Verification items for the finished model (mm, model axes). Give positions to 0.01 mm unless a question says otherwise; leave off trailing zeros. Write each loop counter-clockwise with the first axis right and the second up, starting at its lowest first coordinate (ties: lowest second). Pieces come first, ordered by that corner, then holes.
from build123d import *

# Parameters (mm, degrees)
EXTRUDE_1_DEPTH     = 3
SKETCH_3_R          = 1.25
SKETCH_3_R_2        = 30
SKETCH_3_R_3        = 1.5
CUT_EXTRUDE_1_DEPTH = 3
CUT_EXTRUDE_2_DEPTH = 3
SKETCH_5_R          = 1.25
CUT_EXTRUDE_3_DEPTH = 10


with BuildPart() as part:
    # 草图2 → 凸台-拉伸1 (new body)
    with BuildSketch(Plane(origin=(0, 5, 0), x_dir=(1, 0, 0), z_dir=(0, 1, 0))):
        with BuildLine():
            Line((-250, 28), (0, 43.5))
            ThreePointArc((0, 43.5), (43.5, 0), (0, -43.5))
            Line((0, -43.5), (-250, -28))
            ThreePointArc((-250, -28), (-278, 0), (-250, 28))
        make_face()
    extrude(amount=EXTRUDE_1_DEPTH)

    # 草图3 → 切除-拉伸1 (cut)
    with BuildSketch(Plane(origin=(0, 8, 0), x_dir=(1, 0, 0), z_dir=(0, 1, 0))):
        with Locations(Location((-250, 4, 0), (0, 0, 270))):
            Circle(SKETCH_3_R)
        with Locations(Location((-246, 0, 0), (0, 0, 270))):
            Circle(SKETCH_3_R)
        with Locations(Location((-250, -4, 0), (0, 0, 270))):
            Circle(SKETCH_3_R)
        with Locations(Location((-254, 0, 0), (0, 0, 270))):
            Circle(SKETCH_3_R)
        with Locations(Location((0, 0, 0), (0, 0, 270))):
            Circle(SKETCH_3_R_2)
        with Locations(Location((0, 36.5, 0), (0, 0, 270))):
            Circle(SKETCH_3_R)
        with Locations(Location((12.483735231, 34.298780659, 0), (0, 0, 270))):
            Circle(SKETCH_3_R_3)
        with Locations(Location((23.461747754, 27.960622174, 0), (0, 0, 270))):
            Circle(SKETCH_3_R)
        with Locations(Location((-23.461747754, 27.960622174, 0), (0, 0, 270))):
            Circle(SKETCH_3_R)
        with Locations(Location((-35.945482985, 6.338158485, 0), (0, 0, 270))):
            Circle(SKETCH_3_R)
        with Locations(Location((-35.945482985, -6.338158485, 0), (0, 0, 270))):
            Circle(SKETCH_3_R_3)
        with Locations(Location((-31.609927238, -18.25, 0), (0, 0, 270))):
            Circle(SKETCH_3_R)
        with Locations(Location((-12.483735231, -34.298780659, 0), (0, 0, 270))):
            Circle(SKETCH_3_R)
        with Locations(Location((12.483735231, -34.298780659, 0), (0, 0, 270))):
            Circle(SKETCH_3_R)
        with Locations(Location((23.461747754, -27.960622174, 0), (0, 0, 270))):
            Circle(SKETCH_3_R_3)
        with Locations(Location((31.609927238, -18.25, 0), (0, 0, 270))):
            Circle(SKETCH_3_R)
        with Locations(Location((35.945482985, 6.338158485, 0), (0, 0, 270))):
            Circle(SKETCH_3_R)
        with BuildLine():
            ThreePointArc((-265.553651429, 15.553651429), (-265.553651429, 11.316406256), (-261.316406256, 11.316406256))
            ThreePointArc((-261.316406256, 11.316406256), (-250, 16.003815204), (-238.683593744, 11.316406256))
            ThreePointArc((-238.683593744, 11.316406256), (-234.446348571, 11.316406256), (-234.446348571, 15.553651429))
            ThreePointArc((-234.446348571, 15.553651429), (-250, 21.996184796), (-265.553651429, 15.553651429))
        make_face()
        with BuildLine():
            ThreePointArc((-261.316406256, -11.316406256), (-250, -16.003815204), (-238.683593744, -11.316406256))
            ThreePointArc((-238.683593744, -11.316406256), (-234.446348571, -11.316406256), (-234.446348571, -15.553651429))
            ThreePointArc((-234.446348571, -15.553651429), (-250, -21.996184796), (-265.553651429, -15.553651429))
            ThreePointArc((-265.553651429, -15.553651429), (-265.553651429, -11.316406256), (-261.316406256, -11.316406256))
        make_face()
    extrude(amount=-CUT_EXTRUDE_1_DEPTH, mode=Mode.SUBTRACT)

    # 草图4 → 切除-拉伸2 (cut)
    with BuildSketch(Plane(origin=(0, 8, 0), x_dir=(1, 0, 0), z_dir=(0, 1, 0))):
        with BuildLine():
            Line((-216.23889617, 1.5), (-205.267472927, 20.503062488))
            ThreePointArc((-205.267472927, 20.503062488), (-199.762485666, 21.978119379), (-198.287428775, 16.473132117))
            Line((-198.287428775, 16.473132117), (-206.932170633, 1.5))
            ThreePointArc((-206.932170633, 1.5), (-207.334094422, 0), (-206.932170633, -1.5))
            Line((-206.932170633, -1.5), (-198.287428775, -16.473132117))
            ThreePointArc((-198.287428775, -16.473132117), (-199.762485666, -21.978119379), (-205.267472927, -20.503062488))
            Line((-205.267472927, -20.503062488), (-216.23889617, -1.5))
            ThreePointArc((-216.23889617, -1.5), (-216.640819958, 0), (-216.23889617, 1.5))
        make_face()
        with BuildLine():
            Line((-54.444025551, 1.5), (-65.7023558, 21))
            ThreePointArc((-65.7023558, 21), (-66.800432012, 22.098076211), (-68.300432012, 22.5))
            Line((-68.300432012, 22.5), (-90.81709251, 22.5))
            ThreePointArc((-90.81709251, 22.5), (-92.31709251, 22.098076211), (-93.415168722, 21))
            Line((-93.415168722, 21), (-104.673498971, 1.5))
            ThreePointArc((-104.673498971, 1.5), (-105.075422759, 0), (-104.673498971, -1.5))
            Line((-104.673498971, -1.5), (-93.415168722, -21))
            ThreePointArc((-93.415168722, -21), (-92.31709251, -22.098076211), (-90.81709251, -22.5))
            Line((-90.81709251, -22.5), (-68.300432012, -22.5))
            ThreePointArc((-68.300432012, -22.5), (-66.800432012, -22.098076211), (-65.7023558, -21))
            Line((-65.7023558, -21), (-54.444025551, -1.5))
            ThreePointArc((-54.444025551, -1.5), (-54.042101763, 0), (-54.444025551, 1.5))
        make_face()
        with BuildLine():
            Line((-188.932170633, -1.5), (-180.287428775, -16.473132117))
            ThreePointArc((-180.287428775, -16.473132117), (-181.762485666, -21.978119379), (-187.267472927, -20.503062488))
            Line((-187.267472927, -20.503062488), (-198.23889617, -1.5))
            ThreePointArc((-198.23889617, -1.5), (-198.640819958, 0), (-198.23889617, 1.5))
            Line((-198.23889617, 1.5), (-187.267472927, 20.503062488))
            ThreePointArc((-187.267472927, 20.503062488), (-181.762485666, 21.978119379), (-180.287428775, 16.473132117))
            Line((-180.287428775, 16.473132117), (-188.932170633, 1.5))
            ThreePointArc((-188.932170633, 1.5), (-189.334094422, 0), (-188.932170633, -1.5))
        make_face()
        with BuildLine():
            Line((-170.932170633, -1.5), (-162.287428775, -16.473132117))
            ThreePointArc((-162.287428775, -16.473132117), (-163.762485666, -21.978119379), (-169.267472927, -20.503062488))
            Line((-169.267472927, -20.503062488), (-180.23889617, -1.5))
            ThreePointArc((-180.23889617, -1.5), (-180.640819958, 0), (-180.23889617, 1.5))
            Line((-180.23889617, 1.5), (-169.267472927, 20.503062488))
            ThreePointArc((-169.267472927, 20.503062488), (-163.762485666, 21.978119379), (-162.287428775, 16.473132117))
            Line((-162.287428775, 16.473132117), (-170.932170633, 1.5))
            ThreePointArc((-170.932170633, 1.5), (-171.334094422, 0), (-170.932170633, -1.5))
        make_face()
        with BuildLine():
            Line((-152.932170633, -1.5), (-144.287428775, -16.473132117))
            ThreePointArc((-144.287428775, -16.473132117), (-145.762485666, -21.978119379), (-151.267472927, -20.503062488))
            Line((-151.267472927, -20.503062488), (-162.23889617, -1.5))
            ThreePointArc((-162.23889617, -1.5), (-162.640819958, 0), (-162.23889617, 1.5))
            Line((-162.23889617, 1.5), (-151.267472927, 20.503062488))
            ThreePointArc((-151.267472927, 20.503062488), (-145.762485666, 21.978119379), (-144.287428775, 16.473132117))
            Line((-144.287428775, 16.473132117), (-152.932170633, 1.5))
            ThreePointArc((-152.932170633, 1.5), (-153.334094422, 0), (-152.932170633, -1.5))
        make_face()
        with BuildLine():
            Line((-134.932170633, -1.5), (-126.287428775, -16.473132117))
            ThreePointArc((-126.287428775, -16.473132117), (-127.762485666, -21.978119379), (-133.267472927, -20.503062488))
            Line((-133.267472927, -20.503062488), (-144.23889617, -1.5))
            ThreePointArc((-144.23889617, -1.5), (-144.640819958, 0), (-144.23889617, 1.5))
            Line((-144.23889617, 1.5), (-133.267472927, 20.503062488))
            ThreePointArc((-133.267472927, 20.503062488), (-127.762485666, 21.978119379), (-126.287428775, 16.473132117))
            Line((-126.287428775, 16.473132117), (-134.932170633, 1.5))
            ThreePointArc((-134.932170633, 1.5), (-135.334094422, 0), (-134.932170633, -1.5))
        make_face()
        with BuildLine():
            Line((-116.932170633, -1.5), (-108.287428775, -16.473132117))
            ThreePointArc((-108.287428775, -16.473132117), (-109.762485666, -21.978119379), (-115.267472927, -20.503062488))
            Line((-115.267472927, -20.503062488), (-126.23889617, -1.5))
            ThreePointArc((-126.23889617, -1.5), (-126.640819958, 0), (-126.23889617, 1.5))
            Line((-126.23889617, 1.5), (-115.267472927, 20.503062488))
            ThreePointArc((-115.267472927, 20.503062488), (-109.762485666, 21.978119379), (-108.287428775, 16.473132117))
            Line((-108.287428775, 16.473132117), (-116.932170633, 1.5))
            ThreePointArc((-116.932170633, 1.5), (-117.334094422, 0), (-116.932170633, -1.5))
        make_face()
    extrude(amount=-CUT_EXTRUDE_2_DEPTH, mode=Mode.SUBTRACT)

    # 草图5 → 切除-拉伸3 (cut)
    with BuildSketch(Plane(origin=(0, 8, 0), x_dir=(1, 0, 0), z_dir=(0, 1, 0))):
        with Locations(Location((-44.941689831, 32.96361523, 0), (0, 0, 270))):
            Circle(SKETCH_5_R)
        with Locations(Location((-69.702891128, 31.42842075, 0), (0, 0, 270))):
            Circle(SKETCH_5_R)
        with Locations(Location((-119.225293723, 28.358031789, 0), (0, 0, 270))):
            Circle(SKETCH_5_R)
        with Locations(Location((-94.464092426, 29.89322627, 0), (0, 0, 270))):
            Circle(SKETCH_5_R)
        with Locations(Location((-44.941689831, -32.96361523, 0), (0, 0, 270))):
            Circle(SKETCH_5_R)
        with Locations(Location((-69.702891128, -31.42842075, 0), (0, 0, 270))):
            Circle(SKETCH_5_R)
        with Locations(Location((-94.464092426, -29.89322627, 0), (0, 0, 270))):
            Circle(SKETCH_5_R)
        with Locations(Location((-119.225293723, -28.358031789, 0), (0, 0, 270))):
            Circle(SKETCH_5_R)
    extrude(amount=-CUT_EXTRUDE_3_DEPTH, mode=Mode.SUBTRACT)


solid = part.part
Item 1: Sectioned sample at C-C on y = 6. State how many separate pieces and enclosed holes the cut face has, then the cut area to 3 significant figures.
Answer key:
separate pieces: 1
enclosed holes: 34
area: 14,600 mm2
Item 2: Release check for a two-part mould opening along Z. For faces 1 (the face through (-126.75, 6.48, -35.64)), 2 (the face through (-202.67, 6.52, 8.88)), 3 (the face through (-127.8, 6.5, -22)), 4 (the face through (-115, 8, -1)) record: released by +Z, released by -Z, zero draft, split by the parting line, or undercut.
Answer key:
face 1: released by -Z
face 2: undercut
face 3: undercut
face 4: zero draft
Item 3: Sectioned sample at A-A on x = -80.5. Record the cut outline in (y, z).
Answer key:
outline: (5, -38.51) - (8, -38.51) - (8, -22.5) - (5, -22.5) - close; (5, 22.5) - (8, 22.5) - (8, 38.51) - (5, 38.51) - close
Item 4: Sectioned sample at B-B on x = -225. Record the cut outline in (y, z), then the cut area to 3 significant figures.
Answer key:
outline: (5, -29.55) - (8, -29.55) - (8, 29.55) - (5, 29.55) - close
area: 177 mm2
Item 5: Scan lines: line 1 along Z through (x, y) = (-165, 5.4); line 2 along Z through (x, y) = (0.5, 6.05); line 3 along Z through (x, y) = (-246, 6.8). Record each from-to range of solid material in increasing order.
Answer key:
line 1: z = -33.27 to -22.44, -11.77 to 11.77, 22.44 to 33.27
line 2: z = -43.5 to -37.65, -35.35 to -30, 30 to 43.5
line 3: z = -28.25 to -21.63, -15.5 to -1.25, 1.25 to 15.5, 21.63 to 28.25
Item 6: Depth check by flat-ended pin: pin 1 (1.5 mm diameter, centred on y = 5.5, z = 3, fed in from -X); pin 2 (1.5 mm diameter, centred on x = -85, y = 6.5, fed in from -Z). Enter the tip coordinate at first touch or a pass-through.
Answer key:
pin 1: stops at x = -277.91
pin 2: stops at z = -38.28
